from build123d import *

# Parameters (mm, degrees)
SKETCH_1_W      = 149
SKETCH_1_H      = 138
SKETCH_1_W_2    = 62.5
SKETCH_1_H_2    = 122
EXTRUDE_1_DEPTH = 216
SKETCH_2_W      = 5
SKETCH_2_H      = 20
SKETCH_2_W_2    = 20
SKETCH_2_H_2    = 5
EXTRUDE_2_DEPTH = 5
SKETCH_3_W      = 350
SKETCH_3_H      = 220
EXTRUDE_3_DEPTH = 5
EXTRUDE_START   = 12
EXTRUDE_4_DEPTH = 29
SKETCH_6_W      = 50
SKETCH_6_H      = 20
EXTRUDE_5_DEPTH = 5


with BuildPart() as part:
    # 草图1 → 凸台-拉伸1 (new body)
    with BuildSketch(Plane.XY):
        Rectangle(SKETCH_1_W, SKETCH_1_H)
        with Locations((35.25, 0)):
            Rectangle(SKETCH_1_W_2, SKETCH_1_H_2, mode=Mode.SUBTRACT)
        with Locations((-35.25, 0)):
            Rectangle(SKETCH_1_W_2, SKETCH_1_H_2, mode=Mode.SUBTRACT)
    extrude(amount=EXTRUDE_1_DEPTH)

    # 草图2 → 凸台-拉伸2 (add)
    with BuildSketch(Plane(origin=(0, 0, 0), x_dir=(-1, 0, 0), z_dir=(0, 0, -1))):
        with Locations((72, 0)):
            Rectangle(SKETCH_2_W, SKETCH_2_H)
        with Locations((-72, 0)):
            Rectangle(SKETCH_2_W, SKETCH_2_H)
        with Locations((64.5, 66.5)):
            Rectangle(SKETCH_2_W_2, SKETCH_2_H_2)
        with Locations((-64.5, 66.5)):
            Rectangle(SKETCH_2_W_2, SKETCH_2_H_2)
        with Locations((64.5, -66.5)):
            Rectangle(SKETCH_2_W_2, SKETCH_2_H_2)
        with Locations((-64.5, -66.5)):
            Rectangle(SKETCH_2_W_2, SKETCH_2_H_2)
    extrude(amount=EXTRUDE_2_DEPTH)

    # 草图3 → 凸台-拉伸3 (add)
    with BuildSketch(Plane.XY.offset(216)):
        Rectangle(SKETCH_3_W, SKETCH_3_H)
    extrude(amount=EXTRUDE_3_DEPTH)

    # 草图5 → 凸台-拉伸4 (add)
    with BuildSketch(Plane(origin=(0, 69, 0), x_dir=(1, 0, 0), z_dir=(0, 1, 0)).offset(EXTRUDE_START)):
        Polygon((-146.754147686, -216), (-166.754147686, -196), (-166.754147686, -216), align=None)
        Polygon((117.545852314, -216), (137.545852314, -216), (117.545852314, -196), align=None)
    extrude_4 = extrude(amount=EXTRUDE_4_DEPTH)

    # 草图6 → 凸台-拉伸5 (add)
    with BuildSketch(Plane.XZ.offset(-81)):
        with Locations((142.545852314, 206)):
            Rectangle(SKETCH_6_W, SKETCH_6_H)
        with Locations((-141.754147686, 206)):
            Rectangle(SKETCH_6_W, SKETCH_6_H)
    extrude_5 = extrude(amount=EXTRUDE_5_DEPTH)

    # 镜向1: 凸台-拉伸4, 凸台-拉伸5 across plane
    add(extrude_4.mirror(Plane.ZX))
    add(extrude_5.mirror(Plane.ZX))


solid = part.part
Can you work these out from the model? Positions are in its coordinate system, mm. A direction names the side the tool comes from. Round coordinates to 2 decimals unless told otherwise and drop trailing zeros. Write each loop counter-clockwise with the first axis right and the second up, starting at its lowest first coordinate (ties: lowest second). Pieces come first, ordered by that corner, then holes. Notation, with made-up numbers: M 8,63.25 L 53,63.25 A22 ccw 53,99.25 Z; hole C 30,86.5 d5. An arc over 180 degrees is marked long. Use a Markdown table: item, result.
Item 1: If I drill on line 1 along X through (y, z) = (-55, 85.5); line 2 along Y through (x, z) = (53, 27); line 3 along Z through (x, y) = (39, -55.5), over which ranges is the centre line in solid material (lowest first)? Write a range as [from, to].
Found:
| item | result |
|---|---|
| line 1 | x = [-74.5, -66.5], [-4, 4], [66.5, 74.5] |
| line 2 | y = [-69, -61], [61, 69] |
| line 3 | z = [216, 221] |
Item 2: We'd pull the mould along X, two halves only. Please class faces 4 (the face through (-4, -1, 106)), 5 (the face through (142, -76, 206)), 6 (the face through (74.5, -1, 104)): released by +X, released by -X, zero draft, split by the parting line, or undercut.
Found:
| item | result |
|---|---|
| face 4 | undercut |
| face 5 | zero draft |
| face 6 | released by +X |
Item 3: For pin 1 Ø6 at (y, z) = (-97.5, 210.5) entering from -X; pin 2 Ø2 at (x, z) = (-46, 118) entering from +Y; pin 3 Ø6 at (x, z) = (-135, 205.5) entering from -Y; pin 4 Ø22 at (x, z) = (-131.5, 208) entering from +Y, each with a flat end and sliding along its axis, tell me the tip position at first contact or that it passes through.
Found:
| item | result |
|---|---|
| pin 1 | stops at x = -166.75 |
| pin 2 | stops at y = 69 |
| pin 3 | stops at y = -81 |
| pin 4 | stops at y = 110 |
Item 4: Which directions (+Z, -Z, +X, -X, +Y, -Y) give clear straight access to the entire face, cutting with the end or side of a thin tool? Please do faces 1 (the face through (-36, 1, 216)), 2 (the face through (142, 76, 206)), 3 (the face through (148, 81, 206)).
Found:
| item | result |
|---|---|
| face 1 | -Z |
| face 2 | -Z, +X, -X |
| face 3 | -Z, +X, +Y |
Item 5: I want a section at B-B (y = -33). List the corners of the cut face in (x, z) for me, and give its area (3 significant figures).
Found:
| item | result |
|---|---|
| outline | M -175,216 L -74.5,216 L -74.5,0 L -66.5,0 L -66.5,216 L -4,216 L -4,0 L 4,0 L 4,216 L 66.5,216 L 66.5,0 L 74.5,0 L 74.5,216 L 175,216 L 175,221 L -175,221 Z |
| area | 6,930 mm2 |
Item 6: I want a section at D-D (x = 83). List the corners of the cut face in (y, z) for me.
Found:
| item | result |
|---|---|
| outline | M -110,216 L 110,216 L 110,221 L -110,221 Z |
Item 7: I want a section at A-A (z = 77.5). List the corners of the cut face in (x, y) for me.
Found:
| item | result |
|---|---|
| outline | M -74.5,-69 L 74.5,-69 L 74.5,69 L -74.5,69 Z; hole M -66.5,-61 L -4,-61 L -4,61 L -66.5,61 Z; hole M 4,-61 L 66.5,-61 L 66.5,61 L 4,61 Z |
Item 8: I want a section at C-C (x = 32). List the corners of the cut face in (y, z) for me.
Found:
| item | result |
|---|---|
| outline | M -110,216 L -69,216 L -69,0 L -61,0 L -61,216 L 61,216 L 61,0 L 69,0 L 69,216 L 110,216 L 110,221 L -110,221 Z |
